from build123d import *

# Parameters (mm, degrees)
F1_DEPTH = 50
F2_DEPTH = 10
F3_DEPTH = 20


with BuildPart() as f1:
    # F0 (on Top) → F1 (new body)
    with BuildSketch(Plane.XY):
        with BuildLine():
            ThreePointArc((11.839883195, -9.2096235498), (14.1879922456, -4.8683545514), (15, 0))
            ThreePointArc((15, 0), (14.7213389809, 2.8778774487), (13.8957095187, 5.648827929))
            ThreePointArc((13.8957095187, 5.648827929), (9.2096233049, 11.8398833855), (2.0558258258, 14.858451473))
            ThreePointArc((2.0558258258, 14.858451473), (-5.6488280861, 13.8957094548), (-11.8398831796, 9.2096235695))
            ThreePointArc((-11.8398831796, 9.2096235695), (-14.8584514186, 2.0558262189), (-13.8957094373, -5.6488281293))
            ThreePointArc((-13.8957094373, -5.6488281293), (-9.2096232871, -11.8398833994), (-2.0558259954, -14.8584514495))
            ThreePointArc((-2.0558259954, -14.8584514495), (5.6488280184, -13.8957094824), (11.839883195, -9.2096235498))
        make_face()
    extrude(amount=F1_DEPTH)

    # F0 (on Top) → F2 (join)
    with BuildSketch(Plane.XY):
        with BuildLine():
            ThreePointArc((11.839883195, -9.2096235498), (14.1879922456, -4.8683545514), (15, 0))
            ThreePointArc((15, 0), (14.7213389809, 2.8778774487), (13.8957095187, 5.648827929))
            ThreePointArc((13.8957095187, 5.648827929), (9.2096233049, 11.8398833855), (2.0558258258, 14.858451473))
            ThreePointArc((2.0558258258, 14.858451473), (-5.6488280861, 13.8957094548), (-11.8398831796, 9.2096235695))
            ThreePointArc((-11.8398831796, 9.2096235695), (-14.8584514186, 2.0558262189), (-13.8957094373, -5.6488281293))
            ThreePointArc((-13.8957094373, -5.6488281293), (-9.2096232871, -11.8398833994), (-2.0558259954, -14.8584514495))
            ThreePointArc((-2.0558259954, -14.8584514495), (5.6488280184, -13.8957094824), (11.839883195, -9.2096235498))
        make_face()
        with BuildLine():
            ThreePointArc((13.8957095187, 5.648827929), (14.7213389809, 2.8778774487), (15, 0))
            ThreePointArc((15, 0), (14.1879922456, -4.8683545514), (11.839883195, -9.2096235498))
            Line((11.839883195, -9.2096235498), (17.1570618896, -2.3738633739))
            Line((17.1570618896, -2.3738633739), (13.8957095187, 5.648827929))
        make_face()
        with BuildLine():
            ThreePointArc((2.0558258258, 14.858451473), (9.2096233049, 11.8398833855), (13.8957095187, 5.648827929))
            Line((13.8957095187, 5.648827929), (10.6343569317, 13.6715197637))
            Line((10.6343569317, 13.6715197637), (2.0558258258, 14.858451473))
        make_face()
        with BuildLine():
            Line((6.5227049579, -16.0453831376), (11.839883195, -9.2096235498))
            ThreePointArc((11.839883195, -9.2096235498), (5.6488280184, -13.8957094824), (-2.0558259954, -14.8584514495))
            Line((-2.0558259954, -14.8584514495), (6.5227049579, -16.0453831376))
        make_face()
        with BuildLine():
            ThreePointArc((-11.8398831796, 9.2096235695), (-5.6488280861, 13.8957094548), (2.0558258258, 14.858451473))
            Line((2.0558258258, 14.858451473), (-6.5227049579, 16.0453831376))
            Line((-6.5227049579, 16.0453831376), (-11.8398831796, 9.2096235695))
        make_face()
        with BuildLine():
            Line((-10.6343569317, -13.6715197637), (-2.0558259954, -14.8584514495))
            ThreePointArc((-2.0558259954, -14.8584514495), (-9.2096232871, -11.8398833994), (-13.8957094373, -5.6488281293))
            Line((-13.8957094373, -5.6488281293), (-10.6343569317, -13.6715197637))
        make_face()
        with BuildLine():
            ThreePointArc((-13.8957094373, -5.6488281293), (-14.8584514186, 2.0558262189), (-11.8398831796, 9.2096235695))
            Line((-11.8398831796, 9.2096235695), (-17.1570618896, 2.3738633739))
            Line((-17.1570618896, 2.3738633739), (-13.8957094373, -5.6488281293))
        make_face()
    extrude(amount=F2_DEPTH)

    # F3 (cut): a face of the model
    f3_faces = [f1.faces().sort_by_distance(p)[0] for p in [
        (0, 0, 50),
    ]]
    extrude(f3_faces, amount=-F3_DEPTH, mode=Mode.SUBTRACT)


solid = f1.part
Design review of the part built by this model. Coordinates are the model's own, in mm. A direction names the side the tool comes from. Coordinates: 2 decimals unless noted, no trailing zeros. Order: outer loops, then holes, each group sorted by start corner. A loop starts at its lowest first (then second) coordinate and runs counter-clockwise, first axis right, second up.
Item 1: Take a section at A-A, the plane z = 3. Write out the cut boundary in (x, y), then the cut area to 3 significant figures.
Item 2: For pin 1 Ø3 at (x, z) = (-11, 23.5) entering from +Y; pin 2 Ø1.5 at (x, z) = (1.5, 5) entering from +Y; pin 3 Ø10 at (y, z) = (-5, 25) entering from +X, all flat-tipped, find the tip position at first contact; note any pin that passes through.
Item 3: Take a section at C-C, the plane y = 1.5. Write out the cut boundary in (x, z).
Item 4: For line 1 (Y direction, x = -0.5, z = 24.5); line 2 (X direction, y = 3, z = 28); line 3 (Y direction, x = -11, z = 8.75), list the stretches that pass through material, from the lowest coordinate up.
Item 5: Take a section at B-B, the plane x = 7.5. Write out the cut boundary in (y, z).
Item 6: For faces 1 (the flat face through (9.3, 12.3, 10)), 2 (the flat face through (-9.3, -12.3, 10)), 3 (the flat face through (0, 0, 30)), list the 3-axis set-ups (+Z, -Z, +X, -X, +Y, -Y) from which the entire face can be reached by the end or side of a thin tool; tool diameter is ignored.
Item 7: Take a section at D-D, the plane z = 12.5. Write out the cut boundary in (x, y).
The answers:
1. outline: (-17.16, 2.37) - (-10.63, -13.67) - (6.52, -16.05) - (17.16, -2.37) - (10.63, 13.67) - (-6.52, 16.05) - close
1. area: 779 mm2
2. pin 1: stops at y = 11.61
2. pin 2: stops at y = 15.04
2. pin 3: stops at x = 15
3. outline: (-16.8, 0) - (15.58, 0) - (15.58, 10) - (14.92, 10) - (14.92, 30) - (-14.92, 30) - (-14.92, 10) - (-16.8, 10) - close
4. line 1: y = -14.99 to 14.99
4. line 2: x = -14.7 to 14.7
4. line 3: y = -12.77 to 10.29
5. outline: (-14.79, 0) - (14.11, 0) - (14.11, 10) - (12.99, 10) - (12.99, 30) - (-12.99, 30) - (-12.99, 10) - (-14.79, 10) - close
6. face 1: +Z, +X, +Y
6. face 2: +Z, -X, -Y
6. face 3: +Z, +X, -X, +Y, -Y
7. outline: circle Ø30 at (0, 0)
